Could you check a few things on this drawing? It's one solid part, dimensions in mm from its lowest x, y, z. A direction names the side the tool comes from. Give positions to 0.01 mm unless a question says otherwise; leave off trailing zeros. Order: outer loops, then holes, each group sorted by start corner. A loop starts at its lowest first (then second) coordinate and runs counter-clockwise, first axis right, second up.
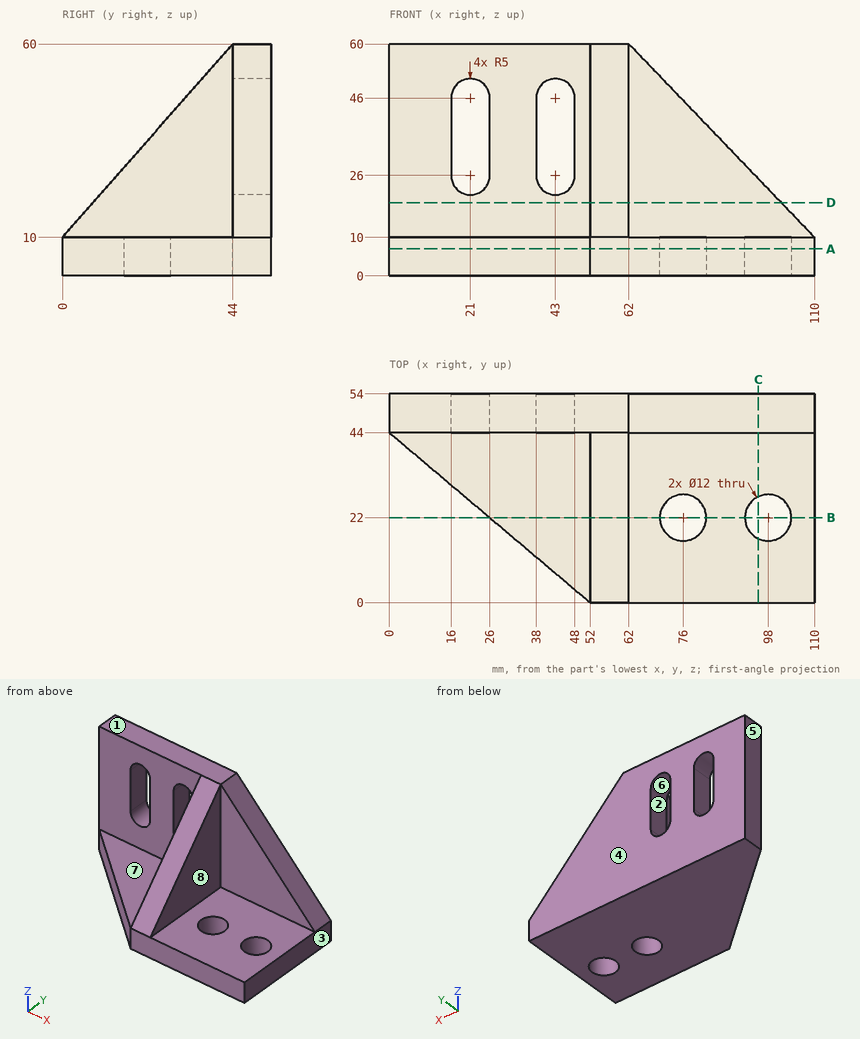
Q1. If we section it at B-B on y = 22: List the corners of the cut face in (x, z) for me.
Filled sheet:
outline: (26, 0) - (70, 0) - (70, 10) - (62, 10) - (62, 35) - (52, 35) - (52, 10) - (26, 10) - close; (82, 0) - (92, 0) - (92, 10) - (82, 10) - close; (104, 0) - (110, 0) - (110, 10) - (104, 10) - close
Q2. Thinking about a two-plate mould opening in X: for the marked faces 1, 2 and 3, which applies, released by +X, released by -X, zero draft, split by the parting line, or undercut?
Filled sheet:
face 1: zero draft
face 2: undercut
face 3: released by +X
Q3. If we section it at A-A on z = 7: List the corners of the cut face in (x, y) for me, plus the area to 3 significant figures.
Filled sheet:
outline: (0, 44) - (52, 0) - (110, 0) - (110, 54) - (0, 54) - close; hole circle Ø12 at (76, 22); hole circle Ø12 at (98, 22)
area: 4,570 mm2
Q4. If we section it at C-C on x = 95.5: List the corners of the cut face in (y, z) for me.
Filled sheet:
outline: (0, 0) - (16.55, 0) - (16.55, 10) - (0, 10) - close; (27.45, 0) - (54, 0) - (54, 25.1) - (44, 25.1) - (44, 10) - (27.45, 10) - close
Q5. I need wall thicknesses on L1, parallel to Y at x = 76, z = 6; L2, parallel to X at y = 21, z = 5.5; L3, parallel to Z at x = 79.5, y = 33.5. Which ranges of each line are inside material? Lowest first, please.
Filled sheet:
L1: y = 0 to 16, 28 to 54
L2: x = 27.18 to 70.08, 81.92 to 92.08, 103.92 to 110
L3: z = 0 to 10
Q6. I'm going to push flat-ended pins straight in: P1, Ø1, axis at y = 32, z = 29.5, coming from the -X side; P2, Ø3, axis at y = 49.5, z = 40.5, coming from the -X side; P3, Ø8, axis at x = 14, z = 52, coming from the -Y side; P4, Ø1, axis at x = 60.5, y = 37, coming from the +Z side. Where does each tip first touch, or does it pass through?
Filled sheet:
P1: stops at x = 52
P2: stops at x = 0
P3: stops at y = 44
P4: stops at z = 52.61
Q7. If we section it at D-D on z = 19: List the corners of the cut face in (x, y) for me.
Filled sheet:
outline: (0, 44) - (52, 44) - (52, 7.92) - (62, 7.92) - (62, 44) - (101.36, 44) - (101.36, 54) - (0, 54) - close
Q8. For the marked faces 4, 5, 6, 7 and 8, which set-ups out of +Z, -Z, +X, -X, +Y, -Y let a thin tool reach every point of the face, with its end or its side?
Filled sheet:
face 4: +Z, -Z, +X, -X, +Y
face 5: +Z, -Z, -X, +Y, -Y
face 6: +Y, -Y
face 7: +Z, -X, -Y
face 8: +Z, +X, -Y
